Work out the finished part from the listing and answer in its coordinate system (mm). Round coordinates to 2 decimals unless told otherwise and drop trailing zeros. Loops run counter-clockwise (first coordinate to the right, second up) from the corner with the lowest first, then second, coordinate; pieces in that order, holes last. Notation, with made-up numbers: M 53,70.25 L 103,70.25 A20 cw 103,103.25 Z; hole C 21.5,26 d1. An arc over 180 degrees is marked long. One line per item, written item: value.
```python
from build123d import *

# Parameters (mm, degrees)
FLANGE_BASE1_DEPTH    = 1.5
ESBO_O7_R             = 2.25
CORTE_EXTRUS_O1_DEPTH = 10
CORTE_EXTRUS_O3_DEPTH = 10
CORTE_EXTRUS_O4_DEPTH = 10


# Sheet-metal steps are written as plain solids
with BuildPart() as part:
    # Esboço2 → Flange-base1 (new body)
    with BuildSketch(Plane.XY):
        Polygon((60, -49.330127019), (-60, -49.330127019), (-88.480762114, 0), (-65, 40.669872981), (65, 40.669872981), (88.480762114, 0), align=None)
    extrude(amount=-FLANGE_BASE1_DEPTH)

    # Esboço7 → Corte-extrusão1 (cut)
    with BuildSketch(Plane(origin=(0, 0, -1.5), x_dir=(-1, 0, 0), z_dir=(0, 0, -1))):
        with Locations((-82.980762114, 0)):
            Circle(ESBO_O7_R)
        with Locations((-55.257737945, -44.330127019)):
            Circle(ESBO_O7_R)
        with Locations((55.257737945, -44.330127019)):
            Circle(ESBO_O7_R)
        with Locations((82.980762114, 0)):
            Circle(ESBO_O7_R)
        with Locations((55.257737945, 35.669872981)):
            Circle(ESBO_O7_R)
        with Locations((-55.257737945, 35.669872981)):
            Circle(ESBO_O7_R)
    extrude(amount=-CORTE_EXTRUS_O1_DEPTH, mode=Mode.SUBTRACT)

    # Esboço8 → Corte-extrusão3 (cut)
    with BuildSketch(Plane.XY):
        with BuildLine():
            Line((-85.980762114, -4.330127019), (-62.5, -45))
            ThreePointArc((-62.5, -45), (-59.330127019, -48.169872981), (-55, -49.330127019))
            Line((-55, -49.330127019), (-88.480762114, -49.330127019))
            Line((-88.480762114, -49.330127019), (-88.480762114, 40.669872981))
            Line((-88.480762114, 40.669872981), (-60, 40.669872981))
            ThreePointArc((-60, 40.669872981), (-64.330127019, 39.509618943), (-67.5, 36.339745962))
            Line((-67.5, 36.339745962), (-85.980762114, 4.330127019))
            ThreePointArc((-85.980762114, 4.330127019), (-87.141016151, 0), (-85.980762114, -4.330127019))
        make_face()
    corte_extrus_o3 = extrude(amount=-CORTE_EXTRUS_O3_DEPTH, mode=Mode.SUBTRACT)

    # Espelhar1: Corte-extrusão3 across plane
    add(corte_extrus_o3.mirror(Plane(origin=(0, 0, 0), x_dir=(0, 0, 1), z_dir=(1, 0, 0))), mode=Mode.SUBTRACT)

    # Esboço9 → Corte-extrusão4 (cut)
    with BuildSketch(Plane.XY):
        with BuildLine():
            Line((-29, -48.330127019), (-29, -46.330127019))
            ThreePointArc((-29, -46.330127019), (-28.707106781, -45.623020238), (-28, -45.330127019))
            Line((-28, -45.330127019), (28, -45.330127019))
            ThreePointArc((28, -45.330127019), (28.707106781, -45.623020238), (29, -46.330127019))
            Line((29, -46.330127019), (29, -48.330127019))
            ThreePointArc((29, -48.330127019), (29.292893219, -49.0372338), (30, -49.330127019))
            Line((30, -49.330127019), (-30, -49.330127019))
            ThreePointArc((-30, -49.330127019), (-29.292893219, -49.0372338), (-29, -48.330127019))
        make_face()
    extrude(amount=-CORTE_EXTRUS_O4_DEPTH, mode=Mode.SUBTRACT)


solid = part.part
```
1) Find the intervals of material crossed by probe 1 along X at (y, z) = (35.5, -1); probe 2 along X at (y, z) = (37.5, -0.15); probe 3 along Y at (x, z) = (16.5, -0.95), in increasing order. Write a range as from..to.
Check values:
probe 1: -67.98..-57.5, -53.01..53.01, 57.5..67.98
probe 2: -66.7..-56.57, -53.95..53.95, 56.57..66.7
probe 3: -45.33..40.67
2) The mould has two halves that part along X. Classify faces 1 (the face through (-64.28, 39.54, -0.74)), 2 (the face through (80.9, -0.86, -0.76)), 3 (the face through (74.405, -24.38, -0.74)), 4 (the face through (-53.6, 37.19, -0.76)): +X half, -X half, draft (parallel to the pull), parting line (faces both ways), or undercut.
Check values:
face 1: -X half
face 2: undercut
face 3: +X half
face 4: undercut
3) Find section C-C (x = 19.5). Give the vertices of the cut face in (y, z).
Check values:
outline: M -45.33,-1.5 L 40.67,-1.5 L 40.67,0 L -45.33,0 Z
4) Find section B-B (z = -0.4). Give the vertices of the cut face in (x, y).
Check values:
outline: M -85.98,-4.33 L -62.5,-45 A8.66 ccw -55,-49.33 L -30,-49.33 A1 ccw -29,-48.33 L -29,-46.33 A1 cw -28,-45.33 L 28,-45.33 A1 cw 29,-46.33 L 29,-48.33 A1 ccw 30,-49.33 L 55,-49.33 A8.66 ccw 62.5,-45 L 85.98,-4.33 A8.66 ccw 85.98,4.33 L 67.5,36.34 A8.66 ccw 60,40.67 L -60,40.67 A8.66 ccw -67.5,36.34 L -85.98,4.33 A8.66 ccw Z; hole C -82.98,0 d4.5; hole C -55.26,-44.33 d4.5; hole C -55.26,35.67 d4.5; hole C 55.26,-44.33 d4.5; hole C 55.26,35.67 d4.5; hole C 82.98,0 d4.5
5) Find section A-A (y = 0). Give the vertices of the cut face in (x, z).
Check values:
outline: M -87.14,-1.5 L -85.23,-1.5 L -85.23,0 L -87.14,0 Z; M -80.73,-1.5 L 80.73,-1.5 L 80.73,0 L -80.73,0 Z; M 85.23,-1.5 L 87.14,-1.5 L 87.14,0 L 85.23,0 Z
6) Each of these flat-tipped pins is pushed along its axis until it touches: pin 1 (7 mm diameter, centred on x = -55.26, y = 35.67, fed in from -Z); pin 2 (0.8 mm diameter, centred on y = -48, z = -1, fed in from +X); pin 3 (0.8 mm diameter, centred on x = 14, z = -0.5, fed in from -Y). Where does it stop, or does it pass through?
Check values:
pin 1: z = -1.5
pin 2: x = 60.19
pin 3: y = -45.33
7) Find section D-D (y = 21). Give the vertices of the cut face in (x, z), then the cut area to 3 significant figures.
Check values:
outline: M -76.36,-1.5 L 76.36,-1.5 L 76.36,0 L -76.36,0 Z
area: 229 mm2
